```python
from build123d import *

# Parameters (mm, degrees)
F0_R     = 67
F1_DEPTH = 2.5
F4_DEPTH = 2
F6_R     = 2.1
F5_R     = 4.75
F5_R_2   = 5.75
F7_DEPTH = 0.501


# Not quite as in the source:
# - the program builds the solid bodies; features that only make, move or delete a surface that nothing else refers to are left out


with BuildPart() as f1:
    # F0 (on Top) → F1 (new body, symmetric)
    with BuildSketch(Plane.XY):
        Circle(F0_R)
    extrude(amount=F1_DEPTH, both=True)

    # F4 (cut): a face of the model
    f4_faces = [f1.faces().sort_by_distance(p)[0] for p in [
        (0, 0, 2.5),
    ]]
    extrude(f4_faces, amount=-F4_DEPTH, mode=Mode.SUBTRACT)

    # F6 (on Top) + F5 (on Top) → F7 (cut, through all)
    with BuildSketch(Plane.XY):
        with Locations((17.5, 8)):
            Circle(F6_R)
        with Locations((-17.5, 8)):
            Circle(F6_R)
    with BuildSketch(Plane.XY):
        Circle(F5_R)
        with Locations((0, -18.75)):
            Circle(F5_R_2)
        with Locations((0, -46.25)):
            Circle(F5_R_2)
    extrude(amount=F7_DEPTH, mode=Mode.SUBTRACT)


solid = f1.part
```
Design review of the part built by this model. Coordinates are the model's own, in mm. A direction names the side the tool comes from. Coordinates: 2 decimals unless noted, no trailing zeros. Write each loop counter-clockwise with the first axis right and the second up, starting at its lowest first coordinate (ties: lowest second). Pieces come first, ordered by that corner, then holes.
1) Machinability: for faces 1 (the flat face through (14, 1, 0.5)), 2 (the flat face through (0, 0, 0)), which of the approach directions +Z, -Z, +X, -X, +Y, -Y give a long, thin tool a straight path to every point of the face, cutting with its end or side? Answer none if there is none.
2) Add section D-D (y = -16.5). Write out the cut boundary in (x, z), plus the area to 3 significant figures.
3) Add section A-A (x = 0). Write out the cut boundary in (y, z), plus the area to 3 significant figures.
4) Mouldability with a two-part tool opening along Y and no side actions: class faces 3 (the flat face through (-1, 1, -2.5)), 4 (the flat face through (0, -19, 0)), 5 (the flat face through (0, -46, 0)), 6 (the cylindrical face through (-14.524, -65.407, -0.979)) as +Y half, -Y half, draft (parallel to the pull), parting line (faces both ways), or undercut.
5) Add section B-B (y = 8). Write out the cut boundary in (x, z).
6) Insertion check: pin 1 (6 mm diameter, centred on x = 0.5, y = -44.5, fed in from +Z). The pin has a flat end and moves straight along its axis. Give the tip position at first contact, or say it passes through.
7) To check wall thickness, follow L1, parallel to Y at x = 0, z = 0.25; L2, parallel to X at y = 8, z = 0.3; L3, parallel to X at y = -46.25, z = 0.45. State the ranges of each line that lie inside material, in increasing order.
8) Add section C-C (z = -0.95). Write out the cut boundary in (x, y).
Check result:
1. face 1: +Z, +X, -X, +Y, -Y
1. face 2: +Z
2. outline: (-64.94, -2.5) - (64.94, -2.5) - (64.94, 0.5) - (5.29, 0.5) - (5.29, 0) - (-5.29, 0) - (-5.29, 0.5) - (-64.94, 0.5) - close
2. area: 384 mm2
3. outline: (-67, -2.5) - (67, -2.5) - (67, 0.5) - (4.75, 0.5) - (4.75, 0) - (-4.75, 0) - (-4.75, 0.5) - (-13, 0.5) - (-13, 0) - (-24.5, 0) - (-24.5, 0.5) - (-40.5, 0.5) - (-40.5, 0) - (-52, 0) - (-52, 0.5) - (-67, 0.5) - close
3. area: 386 mm2
4. face 3: draft
4. face 4: undercut
4. face 5: undercut
4. face 6: parting line
5. outline: (-66.52, -2.5) - (66.52, -2.5) - (66.52, 0.5) - (19.6, 0.5) - (19.6, 0) - (15.4, 0) - (15.4, 0.5) - (-15.4, 0.5) - (-15.4, 0) - (-19.6, 0) - (-19.6, 0.5) - (-66.52, 0.5) - close
6. pin 1: stops at z = 0
7. L1: y = -67 to -52, -40.5 to -24.5, -13 to -4.75, 4.75 to 67
7. L2: x = -66.52 to -19.6, -15.4 to 15.4, 19.6 to 66.52
7. L3: x = -48.48 to -5.75, 5.75 to 48.48
8. outline: circle Ø134 at (0, 0)
